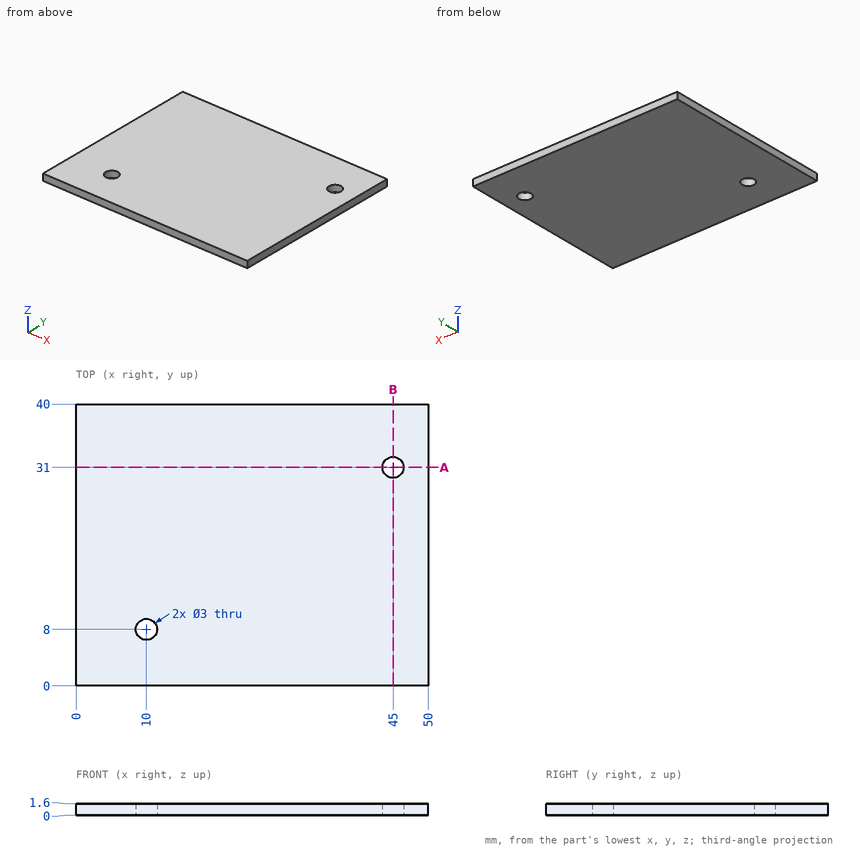
Here's the drawing with two shaded views (mm, measured from the low corner). I have some questions. Coordinates: 2 decimals unless noted, no trailing zeros. Order: outer loops, then holes, each group sorted by start corner. A loop starts at its lowest first (then second) coordinate and runs counter-clockwise, first axis right, second up.
Item 1: If we section it at A-A on y = 31: List the corners of the cut face in (x, z) for me.
Result sheet:
outline: (0, 0) - (43.5, 0) - (43.5, 1.6) - (0, 1.6) - close; (46.5, 0) - (50, 0) - (50, 1.6) - (46.5, 1.6) - close
Item 2: For P1, Ø4, axis at x = 45, y = 31, coming from the +Z side, with a flat end and sliding along its axis, tell me the tip position at first contact or that it passes through.
Result sheet:
P1: stops at z = 1.6
Item 3: I need wall thicknesses on line 1 (X direction, y = 31, z = 1.25); line 2 (Y direction, x = 45, z = 1.25); line 3 (X direction, y = 8, z = 0.35). Which ranges of each line are inside material? Lowest first, please.
Result sheet:
line 1: x = 0 to 43.5, 46.5 to 50
line 2: y = 0 to 29.5, 32.5 to 40
line 3: x = 0 to 8.5, 11.5 to 50
Item 4: If we section it at B-B on x = 45: List the corners of the cut face in (y, z) for me.
Result sheet:
outline: (0, 0) - (29.5, 0) - (29.5, 1.6) - (0, 1.6) - close; (32.5, 0) - (40, 0) - (40, 1.6) - (32.5, 1.6) - close
